from build123d import *

# Parameters (mm, degrees)
SKETCH_1_R           = 2.5
SKETCH_1_R_2         = 13.5
SKETCH_1_R_3         = 4
EXTRUDE_1_DEPTH      = 4
SKETCH_1_3_R         = 13.5
SKETCH_1_3_R_2       = 4
EXTRUDE_2_DEPTH      = 8.5
SKETCH_1_5_R         = 13.5
SKETCH_1_5_R_2       = 4
CUT_EXTRUDE_1_DEPTH  = 1
EXTRUDE_4_DEPTH      = 1
EXTRUDE_4_DEPTH_BACK = 11
SKETCH_2_R           = 6
SKETCH_2_R_2         = 3.975020813
SKETCH_3_R           = 11.5
SKETCH_3_R_2         = 6
CUT_EXTRUDE_2_DEPTH  = 1
FILLET_1_R           = 3
CUT_EXTRUDE_START    = -6.5
SKETCH_3_2_R         = 11.5
SKETCH_3_2_R_2       = 6
CUT_EXTRUDE_3_DEPTH  = 1


with BuildPart() as part:
    # 草图1 → 凸台-拉伸1 (new body)
    # profile 1 of 3: a face of its own
    with BuildSketch(Plane(origin=(0, 0, 0), x_dir=(1, 0, 0), z_dir=(0, 1, 0))):
        with BuildLine():
            Line((4, 24), (-4, 24))
            Line((-4, 24), (-12.309965411, 5.542089098))
            ThreePointArc((-12.309965411, 5.542089098), (0, 13.5), (12.309965411, 5.542089098))
            Line((12.309965411, 5.542089098), (4, 24))
        make_face()
        with Locations(Location((0, 18, 0), (0, 0, 270))):
            Circle(SKETCH_1_R, mode=Mode.SUBTRACT)
    # profile 2 of 3: a face of its own
    with BuildSketch(Plane(origin=(0, 0, 0), x_dir=(1, 0, 0), z_dir=(0, 1, 0))):
        Circle(SKETCH_1_R_2)
        with Locations(Location((0, 0, 0), (0, 0, 270))):
            Circle(SKETCH_1_R_3, mode=Mode.SUBTRACT)
    # profile 3 of 3: a face of its own
    with BuildSketch(Plane(origin=(0, 0, 0), x_dir=(1, 0, 0), z_dir=(0, 1, 0))):
        with BuildLine():
            ThreePointArc((12.309965411, -5.542089098), (0, -13.5), (-12.309965411, -5.542089098))
            Line((-12.309965411, -5.542089098), (-4, -24))
            Line((-4, -24), (4, -24))
            Line((4, -24), (12.309965411, -5.542089098))
        make_face()
        with Locations(Location((0, -18, 0), (0, 0, 270))):
            Circle(SKETCH_1_R, mode=Mode.SUBTRACT)
    extrude(amount=EXTRUDE_1_DEPTH)

    # 草图1<3> → 凸台-拉伸2 (add)
    with BuildSketch(Plane(origin=(0, 0, 0), x_dir=(1, 0, 0), z_dir=(0, 1, 0))):
        with Locations(Location((0, 0, 0), (0, 0, 24.237826184))):
            Circle(SKETCH_1_3_R)
        with Locations(Location((0, 0, 0), (0, 0, 270))):
            Circle(SKETCH_1_3_R_2, mode=Mode.SUBTRACT)
    extrude(amount=EXTRUDE_2_DEPTH)

    # 草图1<5> → 切除-拉伸1 (cut)
    with BuildSketch(Plane(origin=(0, 0, 0), x_dir=(1, 0, 0), z_dir=(0, 1, 0))):
        with Locations(Location((0, 0, 0), (0, 0, 24.237826184))):
            Circle(SKETCH_1_5_R)
        with Locations(Location((0, 0, 0), (0, 0, 270))):
            Circle(SKETCH_1_5_R_2, mode=Mode.SUBTRACT)
    extrude(amount=CUT_EXTRUDE_1_DEPTH, mode=Mode.SUBTRACT)

    # 草图2 → 凸台-拉伸4 (add, two sides: drawn at the far end of the back side and taken through both)
    with BuildSketch(Plane.XZ.offset(-1).offset(-EXTRUDE_4_DEPTH_BACK)):
        with Locations(Location((0, 0, 0), (0, 0, 270))):
            Circle(SKETCH_2_R)
        with Locations(Location((0, 0, 0), (0, 0, 270))):
            Circle(SKETCH_2_R_2, mode=Mode.SUBTRACT)
    extrude(amount=EXTRUDE_4_DEPTH + EXTRUDE_4_DEPTH_BACK)

    # 草图3 → 切除-拉伸2 (cut)
    with BuildSketch(Plane(origin=(0, 8.5, 0), x_dir=(1, 0, 0), z_dir=(0, 1, 0))):
        with Locations(Location((0, 0, 0), (0, 0, 270))):
            Circle(SKETCH_3_R)
        with Locations(Location((0, 0, 0), (0, 0, 90))):
            Circle(SKETCH_3_R_2, mode=Mode.SUBTRACT)
    extrude(amount=-CUT_EXTRUDE_2_DEPTH, mode=Mode.SUBTRACT)

    # 圆角1
    fillet_1_edges = [part.edges().sort_by_distance(p)[0] for p in [
        (-4, 2, -24),
        (4, 2, -24),
        (4, 2, 24),
        (-4, 2, 24),
    ]]
    fillet(fillet_1_edges, radius=FILLET_1_R)

    # 草图3<2> → 切除-拉伸3 (cut)
    with BuildSketch(Plane(origin=(0, 8.5, 0), x_dir=(1, 0, 0), z_dir=(0, 1, 0)).offset(CUT_EXTRUDE_START)):
        with Locations(Location((0, 0, 0), (0, 0, 270))):
            Circle(SKETCH_3_2_R)
        with Locations(Location((0, 0, 0), (0, 0, 90))):
            Circle(SKETCH_3_2_R_2, mode=Mode.SUBTRACT)
    extrude(amount=-CUT_EXTRUDE_3_DEPTH, mode=Mode.SUBTRACT)


solid = part.part
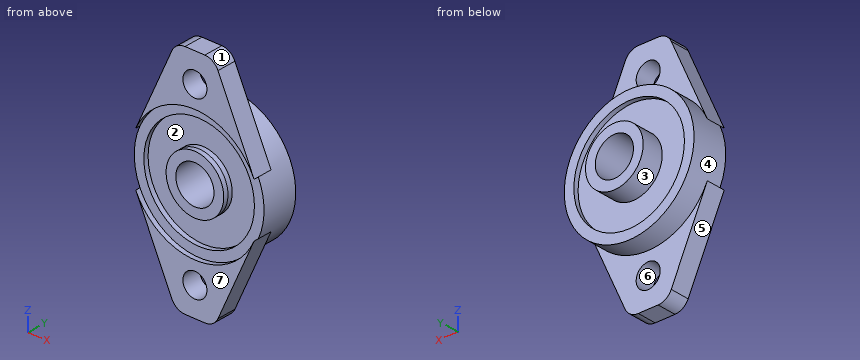
Could you check a few things on this model? Use its own coordinates, in mm. Face numbers are marked on the shaded views. A direction names the side the tool comes from. Round coordinates to 2 decimals unless told otherwise and drop trailing zeros. Order: outer loops, then holes, each group sorted by start corner. A loop starts at its lowest first (then second) coordinate and runs counter-clockwise, first axis right, second up. Notation, with made-up numbers: M 56.5,65.5 L 105.5,65.5 A27 ccw 105.5,96.5 Z; hole C 10,68.25 d8. An arc over 180 degrees is marked long. One line per item, written item: value.
(1) Which directions (+Z, -Z, +X, -X, +Y, -Y) give clear straight access to the entire face, cutting with the end or side of a thin tool? Please do the marked faces 1, 2 and 3.
Ans:
face 1: +Z, +X, +Y, -Y
face 2: -Y
face 3: +Y
(2) I need wall thicknesses on line 1 along X through (y, z) = (8.15, 0); line 2 along X through (y, z) = (4.25, 0); line 3 along X through (y, z) = (9, 0). Which ranges of each line are inside material? Lowest first, please. Write a range as from..to.
Ans:
line 1: x = -13.5..-11.5, -6..-3.98, 3.98..6, 11.5..13.5
line 2: x = -13.5..-3.98, 3.98..13.5
line 3: x = -6..-3.98, 3.98..6
(3) If we mould it in two halves opening along X, with no side actions, what happens to the marked faces 4, 5, 6 and 7? For each: released by +X, released by -X, zero draft, split by the parting line, or undercut.
Ans:
face 4: split by the parting line
face 5: released by -X
face 6: undercut
face 7: zero draft
(4) Imagine slicing it at B-B (y = 8). Write out the boundary of the cut face in (x, z).
Ans:
outline: C 0,0 d27; C 0,0 d12; hole C 0,0 d23; hole C 0,0 d7.95
(5) Imagine slicing it at D-D (x = -5.25). Write out the boundary of the cut face in (y, z).
Ans:
outline: M 0,-21.22 L 4,-21.22 L 4,-12.44 L 8.5,-12.44 L 8.5,-10.23 L 7.5,-10.23 L 7.5,-2.9 L 12,-2.9 L 12,2.9 L 7.5,2.9 L 7.5,10.23 L 8.5,10.23 L 8.5,12.44 L 4,12.44 L 4,21.22 L 0,21.22 L 0,12.44 L 1,12.44 L 1,10.23 L 2,10.23 L 2,2.9 L 0,2.9 L 0,-2.9 L 2,-2.9 L 2,-10.23 L 1,-10.23 L 1,-12.44 L 0,-12.44 Z
(6) I'm going to push flat-ended pins straight in: P1, Ø3, axis at y = 4, z = -16, coming from the -X side; P2, Ø9, axis at x = 0, z = 0, coming from the +Y side; P3, Ø1, axis at y = 7.5, z = -7, coming from the +X side; P4, Ø5.5, axis at x = 4, z = -19, coming from the +Y side. Where does each tip first touch, or does it pass through?
Ans:
P1: stops at x = -8.28
P2: stops at y = 12
P3: stops at x = 11.83
P4: stops at y = 4
(7) Imagine slicing it at C-C (z = 18). Write out the boundary of the cut face in (x, y).
Ans:
outline: M -6.7,0 L -2.5,0 L -2.5,4 L -6.7,4 Z; M 2.5,0 L 6.7,0 L 6.7,4 L 2.5,4 Z
(8) Imagine slicing it at A-A (y = 3.5). Write out the boundary of the cut face in (x, z).
Ans:
outline: M -12.31,-5.54 L -4.8,-22.23 A3 ccw -2.06,-24 L 2.06,-24 A3 ccw 4.8,-22.23 L 12.31,-5.54 A13.5 ccw 12.31,5.54 L 4.8,22.23 A3 ccw 2.06,24 L -2.06,24 A3 ccw -4.8,22.23 L -12.31,5.54 A13.5 ccw Z; hole C 0,0 d7.95; hole C 0,-18 d5; hole C 0,18 d5
